For this review, take the finished solid that the model builds, in its own axes (mm). Face numbers are marked on the shaded views. A direction names the side the tool comes from. Give positions to 0.01 mm unless a question says otherwise; leave off trailing zeros. Loops run counter-clockwise (first coordinate to the right, second up) from the corner with the lowest first, then second, coordinate; pieces in that order, holes last. Notation, with made-up numbers: (10.25, 46.5) - (19.25, 46.5) arc R21 ccw to (19.25, 77.5) - close; hole circle Ø8 at (-11, 17.5). An arc over 180 degrees is marked (long way). Answer in a Markdown table with one row per item.
Autodesk Inventor part; units mm, degrees
ref_plane "Work Plane1" through (104.775, 0, 0) normal (0, 0, -1) x (1, 0, 0)
ref_plane "YZ Plane" through (0, 0, 0) normal (1, 0, 0) x (0, 1, 0)
ref_plane "XZ Plane" through (0, 0, 0) normal (0, 1, 0) x (-1, 0, 0)
sketch "Sketch1" plane through (0, 0, 0) normal (0, 0, 1) x (1, 0, 0)
  line L0 (16, 0) -> (16, 1.5)
  line L1 (16, 1.5) -> (3.36, 1.5)
  line L2 (3.36, 1.5) -> (3.0533, 1.5)
  line L3 (0, 2.77) -> (0, 1.1547)
  line L4 (0, 1.1547) -> (1.1, 1.1547)
  line L5 (1.1, 1.1547) -> (1.7667, 0)
  line L6 (1.7667, 0) -> (16, 0)
  line L7 (0, 2.77) -> (0.59, 2.77)
  line L8 (0.59, 2.77) -> (1.86, 1.5)
  line L9 (3.0533, 1.5) -> (1.86, 1.5)
  line L10 (3.36, 1.5) -> (1.86, 1.5) construction
  line L11 (1.86, 1.5) -> (1.86, 1.5)
  line L12 (-25.4, 0) -> (152.4, 0)
  line L13 (0, -2.1133) -> (0, 12.6797)
  dimension "d0" = 16
  dimension "d1" = 12.64
  dimension "d2" = 1.1
  dimension "d3" = 3
  dimension "d6" = 1.86
  dimension "d7" = 45
  dimension "d8" = 2.3094
  dimension "d9" = 60
  dimension "d10" = 5.54
  dimension "d11" = 3
  dimension "d12" = 0.3067
revolve "Body" add sketch "Sketch1" angle 360 about axis through (1.7667, 0, 0) along (1, 0, 0) contours L6 L5 L4 L3 L7 L8 L9 L2 L1 L0
sketch "Sketch2" plane through (0, 0, 0) normal (-1, 0, 0) x (0, 0, 1)
  circle A0 centre (0, 0) radius 1.1547
  line L0 (0, -6.4055) -> (0, 6.4055)
  line L1 (-6.4055, 0) -> (6.4055, 0)
  line L2 (1.1547, 0) -> (0.5774, -1)
  line L3 (0.5774, -1) -> (-0.5774, -1)
  line L4 (-0.5774, -1) -> (-1.1547, 0)
  line L5 (-1.1547, 0) -> (-0.5774, 1)
  line L6 (-0.5774, 1) -> (0.5774, 1)
  line L7 (0.5774, 1) -> (1.1547, 0)
  point P0 (0, 1.1547)
extrude "Slot" add sketch "Sketch2" against normal up to next contours L7 A0 | A0 L2 | L6 L0 A0 | A0 L0 L3 | L0 L6 A0 | A0 L3 L0 | L4 A0 | A0 L5
thread "Thread"
chamfer "Chamfer1" distance 0.3067 distance2 0.3067 1 edges at (16, -1.5, 0) measured on face at (16, -0.3743, -0.3316)
ref_plane "Work Plane1" through (104.775, 0, 0) normal (0, 0, -1) x (1, 0, 0)
equation "\"d15\" = GEL"
equation "\"d17\" = -0.5 * SPD + 0.5 * GD"
equation "\"d18\" = GUL"
equation "\"d0\" = NLG"
equation "\"d1\" = GEL"
equation "\"d2\" = INTI"
equation "\"d3\" = GD"
equation "\"d6\" = KOH"
equation "\"d7\" = 0.5 * SEWI"
equation "\"d8\" = 1.1547 * SW"
equation "\"d10\" = KOD"
equation "\"d11\" = BDM"
equation "\"d12\" = GAL"
equation "\"NLG\" = 16"
equation "\"INTI\" = 1.1"
equation "\"GEL\" = 12.64"
equation "\"GAL\" = 0.61345 * PTC"
equation "\"KOH\" = 1.86"
equation "\"KOD\" = 5.54"
equation "\"GUL\" = 0.61345 * PTC"
equation "\"SPD\" = NND - 1.2269 * PTC"
equation "\"BDM\" = NND"
equation "\"GD\" = NND"
equation "\"SEWI\" = 90deg"
equation "\"SW\" = 2"
equation "\"TOA\" = 30deg"
equation "\"GD1\" = THREADDIA - 1.2269 * PTC"
equation "\"EPV\" = 3.36"
equation "\"THREADDIA\" = 3"
equation "\"PTC\" = 0.5"
equation "\"NND\" = 3"
equation "\"E0\" = 2.31"
properties part number "ISO 10642  - M3  x  16" material "Steel"
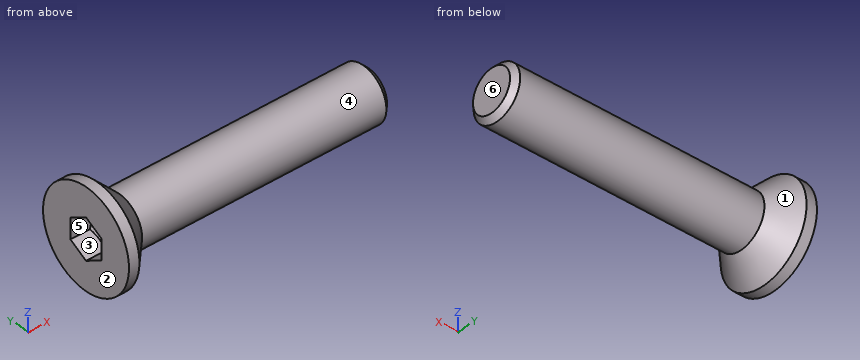
1. For the marked faces 4, 5 and 6, list the 3-axis set-ups (+Z, -Z, +X, -X, +Y, -Y) from which the entire face can be reached by the end or side of a thin tool; tool diameter is ignored.
Values:
| item | result |
|---|---|
| face 4 | +X |
| face 5 | -X |
| face 6 | +Z, -Z, +X, +Y, -Y |
2. Mouldability with a two-part tool opening along Z and no side actions: class the marked faces 1, 2 and 3 as released by +Z, released by -Z, zero draft, split by the parting line, or undercut.
Values:
| item | result |
|---|---|
| face 1 | split by the parting line |
| face 2 | zero draft |
| face 3 | undercut |
3. Clearance check with flat-ended pins moving along their axes: pin 1 (2 mm diameter, centred on y = 1, z = 1, fed in from +X); pin 2 (3 mm diameter, centred on x = 13, y = -0.5, fed in from -Z); pin 3 (1 mm diameter, centred on x = 1.5, y = 0, fed in from -Z); pin 4 (1.5 mm diameter, centred on x = 10.5, z = 1, fed in from +Y). State where each tip first meets the part, or that it passes through.
Values:
| item | result |
|---|---|
| pin 1 | stops at x = 16 |
| pin 2 | stops at z = -1.5 |
| pin 3 | stops at z = -2.36 |
| pin 4 | stops at y = 1.48 |
4. Wall thickness on line 1 (Y direction, x = 14.75, z = 0.65); line 2 (Z direction, x = 4.75, y = 1.25); line 3 (Z direction, x = 14.5, y = -0.25): over which ranges is each line inside the solid? List them lowest first. Write a range as [from, to].
Values:
| item | result |
|---|---|
| line 1 | y = [-1.35, 1.35] |
| line 2 | z = [-0.83, 0.83] |
| line 3 | z = [-1.48, 1.48] |
5. We need section A-A, the plane x = 9. Give the boundary of the cut face in (y, z), and give its area (3 significant figures).
Values:
| item | result |
|---|---|
| outline | circle Ø3 at (0, 0) |
| area | 7.07 mm^2 |
